from build123d import *

# Parameters (mm, degrees)
SKETCH1_R                = 12.5
BOSS_EXTRUDE1_DEPTH      = 60
BOSS_EXTRUDE1_DEPTH_BACK = 60
SKETCH2_R                = 4
BOSS_EXTRUDE2_DEPTH      = 7
SKETCH3_R                = 4
BOSS_EXTRUDE3_DEPTH      = 7


with BuildPart() as part:
    # Sketch1 → Boss-Extrude1 (new body, two sides)
    with BuildSketch(Plane(origin=(0, 0, 0), x_dir=(1, 0, 0), z_dir=(0, 1, 0))) as boss_extrude1_sk:
        Circle(SKETCH1_R)
    extrude(amount=BOSS_EXTRUDE1_DEPTH)
    extrude(boss_extrude1_sk.sketch, amount=-BOSS_EXTRUDE1_DEPTH_BACK)

    # Sketch2 → Boss-Extrude2 (add)
    with BuildSketch(Plane(origin=(0, 60, 0), x_dir=(1, 0, 0), z_dir=(0, 1, 0))):
        Circle(SKETCH2_R)
    extrude(amount=BOSS_EXTRUDE2_DEPTH)

    # Sketch3 → Boss-Extrude3 (add)
    with BuildSketch(Plane.XZ.offset(60)):
        Circle(SKETCH3_R)
    extrude(amount=BOSS_EXTRUDE3_DEPTH)


solid = part.part
Source: CAD feature listing. Evaluate the final solid. Frame: model axes, mm. A direction names the side the tool comes from. Give positions to 0.01 mm unless a question says otherwise; leave off trailing zeros. Order: outer loops, then holes, each group sorted by start corner. A loop starts at its lowest first (then second) coordinate and runs counter-clockwise, first axis right, second up. Notation, with made-up numbers: (-4, 52) -> (15, 52) arc R29 cw to (15, 83) -> close; hole circle Ø6 at (-3.5, 50). An arc over 180 degrees is marked (long way). Write item = value, one per line.
Item 1: Section query C-C (y = -29). Output: boundary loops of the cut face in (x, z).
Check result:
outline = circle Ø25 at (0, 0)
Item 2: Contact query for flat-ended pins moving along their axis: pin 1 (3 mm diameter, centred on y = 43.5, z = -3, fed in from +X); pin 2 (1.5 mm diameter, centred on y = 14.5, z = 5.5, fed in from -X); pin 3 (12 mm diameter, centred on x = -9, z = 9, fed in from +Y). Output: stop coordinate, or through.
Check result:
pin_1 = 12.41
pin_2 = -11.56
pin_3 = 60
Item 3: Section query B-B (z = 0). Output: boundary loops of the cut face in (x, y).
Check result:
outline = (-12.5, -60) -> (-4, -60) -> (-4, -67) -> (4, -67) -> (4, -60) -> (12.5, -60) -> (12.5, 60) -> (4, 60) -> (4, 67) -> (-4, 67) -> (-4, 60) -> (-12.5, 60) -> close
Item 4: Set-up query: faces 1 (the face through (-0.867, -63.451, -3.905)), 2 (the face through (11.923, 0.84, -3.755)), 3 (the face through (-3, 60, -3)). Return all of +Z, -Z, +X, -X, +Y, -Y with unobstructed straight access to the full face (end or side cutting, diameter ignored); none if empty.
Check result:
face_1 = -Y
face_2 = +Y, -Y
face_3 = +Y
Item 5: Section query D-D (x = -7.5). Output: boundary loops of the cut face in (y, z), then the cut area to 3 significant figures.
Check result:
outline = (-60, -10) -> (60, -10) -> (60, 10) -> (-60, 10) -> close
area = 2,400 mm²
Item 6: Ray query, probe 1 along Y at (x, z) = (4.5, 1.75); probe 2 along Z at (x, y) = (-0.25, 37); probe 3 along Z at (x, y) = (-3.5, -43). Return the intervals inside material, ascending.
Check result:
probe_1 = -60 to 60
probe_2 = -12.5 to 12.5
probe_3 = -12 to 12
Item 7: Section query A-A (x = 0). Output: boundary loops of the cut face in (y, z).
Check result:
outline = (-67, -4) -> (-60, -4) -> (-60, -12.5) -> (60, -12.5) -> (60, -4) -> (67, -4) -> (67, 4) -> (60, 4) -> (60, 12.5) -> (-60, 12.5) -> (-60, 4) -> (-67, 4) -> close
